The drawing under review shows one solid part. Ordinate dimensions are in mm from its lowest x, y, z. A direction names the side the tool comes from. Round coordinates to 2 decimals unless told otherwise and drop trailing zeros. Write each loop counter-clockwise with the first axis right and the second up, starting at its lowest first coordinate (ties: lowest second). Pieces come first, ordered by that corner, then holes.
Item 1: Draft analysis for pull direction Y (two halves, no side actions). For the marked faces 1, 2 and 3, state which applies: +Y half, -Y half, draft (parallel to the pull), parting line (faces both ways), or undercut.
Item 2: Add section B-B (y = 15.5). Give the boundary of the cut face in (x, z).
Item 3: Add section A-A (z = 25). Give the boundary of the cut face in (x, y).
Item 4: Add section C-C (x = 21). Give the boundary of the cut face in (y, z), plus the area to 3 significant figures.
Item 5: Machinability: for the marked faces 4 and 5, which of the approach directions +Z, -Z, +X, -X, +Y, -Y give a long, thin tool a straight path to every point of the face, cutting with its end or side? Answer none if there is none.
Item 6: To check wall thickness, follow L1, parallel to X at y = 17.5, z = 24.5; L2, parallel to Y at x = 12, z = 18.5; L3, parallel to X at y = 40, z = 2.5. State the ranges of each line that lie inside material, in increasing order.
Item 7: Add section D-D (y = 24). State how many separate pieces and enclosed holes the cut face has.
Item 8: Clearance check with flat-ended pins moving along their axes: pin 1 Ø8 at (x, z) = (5.5, 23) entering from +Y; pin 2 Ø5 at (x, z) = (44, 28.5) entering from -Y; pin 3 Ø4 at (x, y) = (18, 30) entering from -Z; pin 4 Ø2.5 at (x, y) = (34.32, 23.16) entering from +Z. State where each tip first meets the part, or that it passes through.
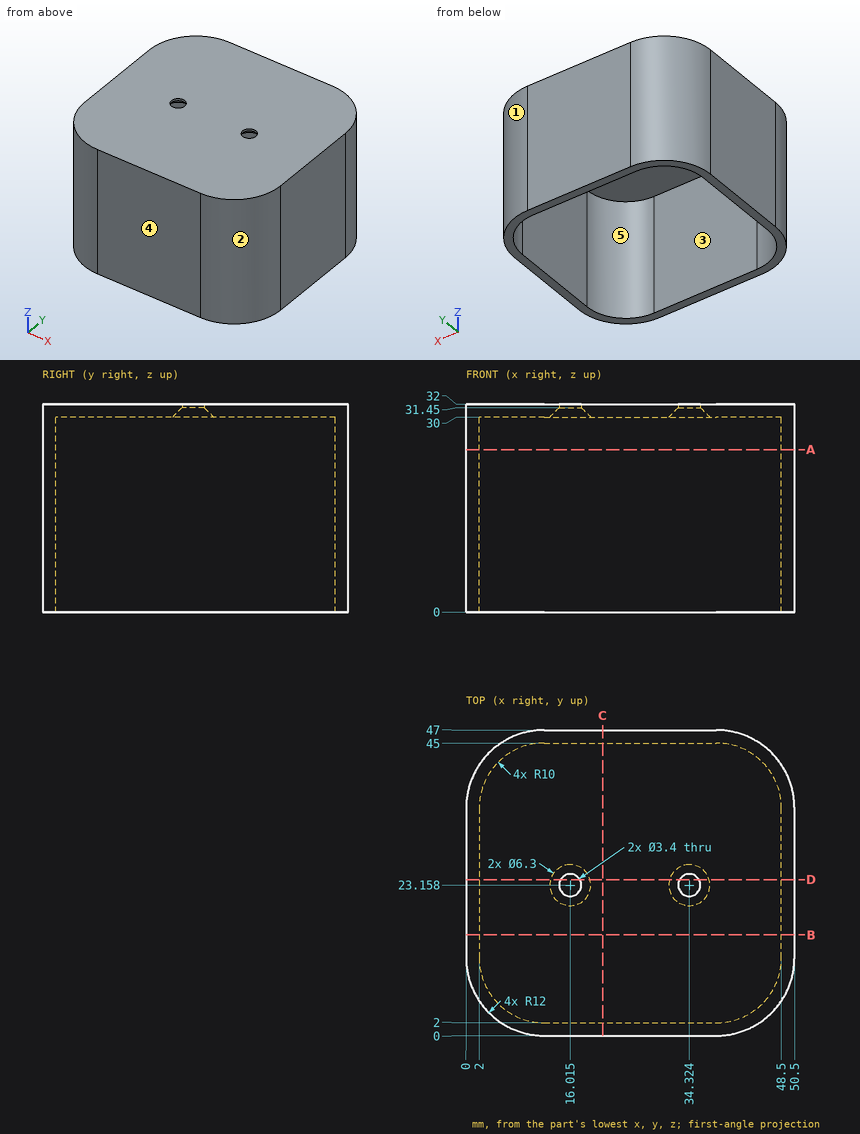
Numbers:
1. face 1: +Y half
1. face 2: -Y half
1. face 3: undercut
2. outline: (0, 0) - (2, 0) - (2, 30) - (48.5, 30) - (48.5, 0) - (50.5, 0) - (50.5, 32) - (0, 32) - close
3. outline: (0, 12) arc R12 ccw to (12, 0) - (38.5, 0) arc R12 ccw to (50.5, 12) - (50.5, 35) arc R12 ccw to (38.5, 47) - (12, 47) arc R12 ccw to (0, 35) - close; hole (2, 12) arc R10 ccw to (12, 2) - (38.5, 2) arc R10 ccw to (48.5, 12) - (48.5, 35) arc R10 ccw to (38.5, 45) - (12, 45) arc R10 ccw to (2, 35) - close
4. outline: (0, 0) - (2, 0) - (2, 30) - (45, 30) - (45, 0) - (47, 0) - (47, 32) - (0, 32) - close
4. area: 214 mm2
5. face 4: +Z, -Z, +X, -X, -Y
5. face 5: -Z
6. L1: x = 0 to 2, 48.5 to 50.5
6. L2: y = 0 to 2, 45 to 47
6. L3: x = 1.09 to 3.34, 47.16 to 49.41
7. separate pieces: 3
7. enclosed holes: 0
8. pin 1: stops at y = 46.74
8. pin 2: stops at y = 0.38
8. pin 3: stops at z = 30
8. pin 4: passes through
